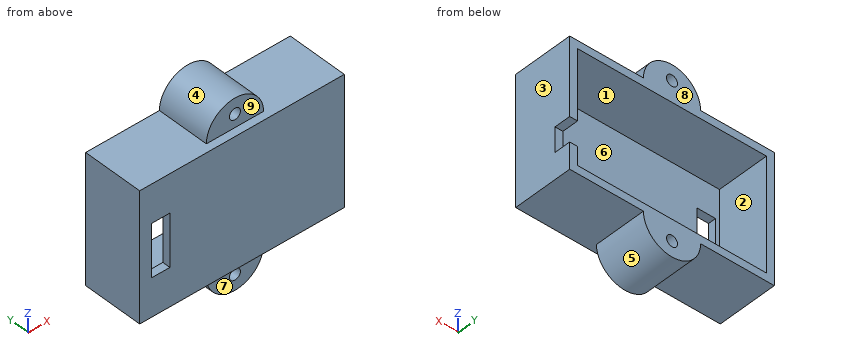
from build123d import *

# Parameters (mm, degrees)
SKETCH1_R           = 2.1
SKETCH1_W           = 72
SKETCH1_H           = 43
BOSS_EXTRUDE1_DEPTH = 20
SKETCH2_W           = 78
SKETCH2_H           = 49
BOSS_EXTRUDE2_DEPTH = 3
SKETCH3_W           = 7
SKETCH3_H           = 20
CUT_EXTRUDE1_DEPTH  = 10
SKETCH4_W           = 9.4
SKETCH4_H           = 6.25
CUT_EXTRUDE2_DEPTH  = 10


with BuildPart() as part:
    # Sketch1 → Boss-Extrude1 (new body)
    with BuildSketch(Plane(origin=(0, 0, 0), x_dir=(1, 0, 0), z_dir=(0, 1, 0))):
        with BuildLine():
            Line((-39, 24.5), (-39, 10.886061931))
            Line((-39, 10.886061931), (-39, -10.886061931))
            Line((-39, -10.886061931), (-39, -24.5))
            Line((-39, -24.5), (-10.89, -24.5))
            ThreePointArc((-10.89, -24.5), (0, -35.39), (10.89, -24.5))
            Line((10.89, -24.5), (39, -24.5))
            Line((39, -24.5), (39, -10.886061931))
            Line((39, -10.886061931), (39, 10.886061931))
            Line((39, 10.886061931), (39, 24.5))
            Line((39, 24.5), (10.89, 24.5))
            ThreePointArc((10.89, 24.5), (0, 35.39), (-10.89, 24.5))
            Line((-10.89, 24.5), (-39, 24.5))
        make_face()
        with Locations(Location((0, -29.5, 0), (0, 0, 270))):
            Circle(SKETCH1_R, mode=Mode.SUBTRACT)
        with Locations(Location((0, 29.5, 0), (0, 0, 270))):
            Circle(SKETCH1_R, mode=Mode.SUBTRACT)
        Rectangle(SKETCH1_W, SKETCH1_H, mode=Mode.SUBTRACT)
    extrude(amount=BOSS_EXTRUDE1_DEPTH)

    # Sketch2 → Boss-Extrude2 (add)
    with BuildSketch(Plane.XZ):
        Rectangle(SKETCH2_W, SKETCH2_H)
    extrude(amount=BOSS_EXTRUDE2_DEPTH)

    # Sketch3 → Cut-Extrude1 (cut)
    with BuildSketch(Plane(origin=(0, 0, 0), x_dir=(1, 0, 0), z_dir=(0, 1, 0))):
        with Locations((-31, 0)):
            Rectangle(SKETCH3_W, SKETCH3_H)
    extrude(amount=-CUT_EXTRUDE1_DEPTH, mode=Mode.SUBTRACT)

    # Sketch4 → Cut-Extrude2 (cut)
    with BuildSketch(Plane(origin=(39, 0, 0), x_dir=(0, 0, -1), z_dir=(1, 0, 0))):
        with Locations((9.8, 16.875)):
            Rectangle(SKETCH4_W, SKETCH4_H)
    extrude(amount=-CUT_EXTRUDE2_DEPTH, mode=Mode.SUBTRACT)


solid = part.part
The model under review builds one solid part; all positions refer to its coordinate system, in mm. Face numbers are marked on the shaded views. A direction names the side the tool comes from. Round coordinates to 2 decimals unless told otherwise and drop trailing zeros. Order: outer loops, then holes, each group sorted by start corner. A loop starts at its lowest first (then second) coordinate and runs counter-clockwise, first axis right, second up. Notation, with made-up numbers: (-24, -39) -> (-19, -39) arc R16 cw to (-19, -24) -> close; hole circle Ø6 at (-5, -28). An arc over 180 degrees is marked (long way). Return JSON: item names as keys, results as strings.
1. The part is to be moulded in two halves that separate along X. For the marked faces 1, 2, 3 and 4, say which applies: +X half, -X half, draft (parallel to the pull), parting line (faces both ways), or undercut.
Answer block:
{"face 1": "undercut", "face 2": "undercut", "face 3": "+X half", "face 4": "parting line"}
2. Take a section at D-D (z = -29.5). Write out the cut boundary in (x, y).
Answer block:
{"outline": "(-9.67, 0) -> (-2.1, 0) -> (-2.1, 20) -> (-9.67, 20) -> close; (2.1, 0) -> (9.67, 0) -> (9.67, 20) -> (2.1, 20) -> close"}
3. Take a section at A-A (x = 0). Write out the cut boundary in (y, z), then the cut area to 3 significant figures.
Answer block:
{"outline": "(-3, -24.5) -> (0, -24.5) -> (0, -27.4) -> (20, -27.4) -> (20, -21.5) -> (0, -21.5) -> (0, 21.5) -> (20, 21.5) -> (20, 27.4) -> (0, 27.4) -> (0, 24.5) -> (-3, 24.5) -> close; (0, -35.39) -> (20, -35.39) -> (20, -31.6) -> (0, -31.6) -> close; (0, 31.6) -> (20, 31.6) -> (20, 35.39) -> (0, 35.39) -> close", "area": "535 mm²"}
4. For the marked faces 5, 6, 7, 8 and 9, list the 3-axis set-ups (+Z, -Z, +X, -X, +Y, -Y) from which the entire face can be reached by the end or side of a thin tool; tool diameter is ignored.
Answer block:
{"face 5": "-Z, +Y, -Y", "face 6": "+Y", "face 7": "-Z, +X, -X, -Y", "face 8": "+Z, -Z, +X, -X, +Y", "face 9": "+Z, +X, -X, -Y"}
5. Insertion check: P1, Ø0.9, axis at x = 38, y = 17.5, coming from the +Z side; P2, Ø1, axis at x = -23, z = 26, coming from the +Y side; P3, Ø12, axis at x = -0.5, z = 31, coming from the -Y side; P4, Ø7, axis at x = 4.5, y = 6.5, coming from the -Z side. Each pin has a flat end and moves straight along its axis. Give the tip position at first contact, or say it passes through.
Answer block:
{"P1": "stops at z = 24.5", "P2": "passes through", "P3": "stops at y = 0", "P4": "stops at z = -35.34"}
6. Take a section at C-C (z = 13). Write out the cut boundary in (x, y), then the cut area to 3 significant figures.
Answer block:
{"outline": "(-39, -3) -> (39, -3) -> (39, 20) -> (36, 20) -> (36, 0) -> (-36, 0) -> (-36, 20) -> (-39, 20) -> close", "area": "354 mm²"}
7. For L1, parallel to X at y = 8.5, z = 19; L2, parallel to Z at x = -12.5, y = 2.25; L3, parallel to Z at x = 3, y = 6.5, list the stretches that pass through material, from the lowest coordinate up. Write a range as [from, to].
Answer block:
{"L1": "x = [-39, -36], [36, 39]", "L2": "z = [-24.5, -21.5], [21.5, 24.5]", "L3": "z = [-34.97, -21.5], [21.5, 34.97]"}
8. Take a section at B-B (y = 7.75). Write out the cut boundary in (x, z), then the cut area to 3 significant figures.
Answer block:
{"outline": "(-39, -24.5) -> (-10.89, -24.5) arc R10.89 ccw to (10.89, -24.5) -> (39, -24.5) -> (39, 24.5) -> (10.89, 24.5) arc R10.89 ccw to (-10.89, 24.5) -> (-39, 24.5) -> close; hole (-36, -21.5) -> (36, -21.5) -> (36, 21.5) -> (-36, 21.5) -> close; hole circle Ø4.2 at (0, -29.5); hole circle Ø4.2 at (0, 29.5)", "area": "1,070 mm²"}
